Input: part model. Units: mm. Frame: model coordinates. A direction names the side the tool comes from. Coordinates: 2 decimals unless noted, no trailing zeros. Order: outer loops, then holes, each group sorted by start corner. A loop starts at its lowest first (then second) coordinate and runs counter-clockwise, first axis right, second up. Notation, with made-up numbers: M 38.5,74 L 96.5,74 A16 ccw 96.5,78 Z; hole C 17,2.5 d8. An arc over 180 degrees is marked long. One line per item, written item: value.
```python
from build123d import *

# Parameters (mm, degrees)
BOSS_EXTRUDE2_DEPTH   = 2.5
BOSS_EXTRUDE2_2_DEPTH = 2.5
BOSS_EXTRUDE2_3_DEPTH = 2.5
BOSS_EXTRUDE2_4_DEPTH = 2.5
BOSS_EXTRUDE3_DEPTH   = 1.5
SKETCH1_W             = 10
SKETCH1_H             = 10
BOSS_EXTRUDE4_DEPTH   = 2.8
CUT_EXTRUDE11_DEPTH   = 1
CUT_EXTRUDE14_DEPTH   = 1


with BuildPart() as part:
    # Sketch2 → Boss-Extrude2 (new body)
    with BuildSketch(Plane(origin=(0, 0, 0), x_dir=(1, 0, 0), z_dir=(0, 1, 0))):
        Polygon((-2, 6), (-6, 6), (-6, 2), (-5, 2), (-5, 5), (-2, 5), align=None)
    extrude(amount=BOSS_EXTRUDE2_DEPTH)



with BuildPart() as body_2:
    # Sketch2 → Boss-Extrude2 2 (new body)
    with BuildSketch(Plane(origin=(0, 0, 0), x_dir=(1, 0, 0), z_dir=(0, 1, 0))):
        Polygon((2, 6), (2, 5), (5, 5), (5, 2), (6, 2), (6, 6), align=None)
    extrude(amount=BOSS_EXTRUDE2_2_DEPTH)


with BuildPart() as body_3:
    # Sketch2 → Boss-Extrude2 3 (new body)
    with BuildSketch(Plane(origin=(0, 0, 0), x_dir=(1, 0, 0), z_dir=(0, 1, 0))):
        Polygon((5, -2), (5, -5), (2, -5), (2, -6), (6, -6), (6, -2), align=None)
    extrude(amount=BOSS_EXTRUDE2_3_DEPTH)


with BuildPart() as body_4:
    # Sketch2 → Boss-Extrude2 4 (new body)
    with BuildSketch(Plane(origin=(0, 0, 0), x_dir=(1, 0, 0), z_dir=(0, 1, 0))):
        Polygon((-6, -2), (-5, -2), (-5, -5), (-2, -5), (-2, -6), (-6, -6), align=None)
    extrude(amount=BOSS_EXTRUDE2_4_DEPTH)

    # Sketch2<4> → Boss-Extrude3 (add)
    with BuildSketch(Plane(origin=(0, 0, 0), x_dir=(1, 0, 0), z_dir=(0, 1, 0))):
        Polygon((-2, 6), (-6, 6), (-6, 2), (-5, 2), (-5, 5), (-2, 5), align=None)
        Polygon((2, 6), (2, 5), (5, 5), (5, 2), (6, 2), (6, 6), align=None)
        Polygon((5, -2), (5, -5), (2, -5), (2, -6), (6, -6), (6, -2), align=None)
        Polygon((-6, -2), (-5, -2), (-5, -5), (-2, -5), (-2, -6), (-6, -6), align=None)
    extrude(amount=-BOSS_EXTRUDE3_DEPTH)


with BuildPart() as boss_extrude3_piece_1:
    # of the separate pieces the step leaves, piece 1, a body of its own (boss_extrude3_pieces)
    add(body_4.part.solids().sort_by_distance((-6, 2.5, 2))[0])


with BuildPart() as boss_extrude3_piece_2:
    # of the separate pieces the step leaves, piece 2, a body of its own (boss_extrude3_pieces)
    add(body_4.part.solids().sort_by_distance((-2, 0, -6))[0])


with BuildPart() as boss_extrude3_piece_3:
    # of the separate pieces the step leaves, piece 3, a body of its own (boss_extrude3_pieces)
    add(body_4.part.solids().sort_by_distance((2, 0, -6))[0])


with BuildPart() as boss_extrude3_piece_4:
    # of the separate pieces the step leaves, piece 4, a body of its own (boss_extrude3_pieces)
    add(body_4.part.solids().sort_by_distance((5, 0, 2))[0])


with BuildPart() as part_1:
    add(part.part)

    add(body_2.part)  # Boss-Extrude4 merges body 2

    add(body_3.part)  # Boss-Extrude4 merges body 3

    add(boss_extrude3_piece_1.part)  # Boss-Extrude4 merges Boss-Extrude3 piece 1

    add(boss_extrude3_piece_2.part)  # Boss-Extrude4 merges Boss-Extrude3 piece 2

    add(boss_extrude3_piece_3.part)  # Boss-Extrude4 merges Boss-Extrude3 piece 3

    add(boss_extrude3_piece_4.part)  # Boss-Extrude4 merges Boss-Extrude3 piece 4
    # Sketch1 → Boss-Extrude4 (add)
    with BuildSketch(Plane(origin=(0, 0, 0), x_dir=(1, 0, 0), z_dir=(0, 1, 0))):
        Rectangle(SKETCH1_W, SKETCH1_H)
        with BuildLine():
            ThreePointArc((1.617598637, -1.615265837), (3.065, 0), (1.617598637, 1.615265837))
            ThreePointArc((1.617598637, 1.615265837), (1.474163525, 1.620673027), (1.331431871, 1.605489361))
            Line((1.331431871, 1.605489361), (-1.677221968, 1.064808042))
            ThreePointArc((-1.677221968, 1.064808042), (-1.895132853, 0.999347796), (-2.092605578, 0.886322491))
            ThreePointArc((-2.092605578, 0.886322491), (-2.54112078, 0), (-2.092605578, -0.886322491))
            ThreePointArc((-2.092605578, -0.886322491), (-1.895132853, -0.999347796), (-1.677221968, -1.064808042))
            Line((-1.677221968, -1.064808042), (1.331431871, -1.605489361))
            ThreePointArc((1.331431871, -1.605489361), (1.474163525, -1.620673027), (1.617598637, -1.615265837))
        make_face(mode=Mode.SUBTRACT)
    extrude(amount=BOSS_EXTRUDE4_DEPTH)

    # 3DSketch1 → Cut-Extrude11 (cut, along a direction that is not the sketch's normal)
    with BuildSketch(Plane(origin=(5, 2.8, 5), x_dir=(-0.693702510890827, -0.1937876486453734, -0.6937025108908424), z_dir=(0.7071067811865555, 0, -0.7071067811865397))):
        Polygon((0, 0), (-0.732362778, 3.707562105), (7.206933902, 0), align=None)
    extrude(amount=-CUT_EXTRUDE11_DEPTH, dir=(1, 0, 0), mode=Mode.SUBTRACT)

    # 3DSketch1<9> → Cut-Extrude14 (cut, along a direction that is not the sketch's normal)
    with BuildSketch(Plane(origin=(5, 2.8, 5), x_dir=(-0.693702510890827, -0.1937876486453734, -0.6937025108908424), z_dir=(0.7071067811865555, 0, -0.7071067811865397))):
        Polygon((0, 0), (-0.732362778, 3.707562105), (7.206933902, 0), align=None)
    extrude(amount=CUT_EXTRUDE14_DEPTH, dir=(0, 0, -1), mode=Mode.SUBTRACT)


solid = part_1.part
```
(1) Cut plane A-A on y = 0.5. Output: boundary loops of the cut face in (x, z) (3 decimals).
Data:
outline: M -6,-6 L -2,-6 L -2,-5 L 2,-5 L 2,-6 L 6,-6 L 6,-2 L 5,-2 L 5,2 L 6,2 L 6,6 L 2,6 L 2,5 L -2,5 L -2,6 L -6,6 L -6,2 L -5,2 L -5,-2 L -6,-2 Z; hole M -2.093,-0.886 A1 ccw -1.677,-1.065 L 1.331,-1.605 A1 ccw 1.618,-1.615 A1.625 ccw 1.618,1.615 A1 ccw 1.331,1.605 L -1.677,1.065 A1 ccw -2.093,0.886 A1.1 ccw Z
(2) First-contact query: pin 1 (5 mm diameter, centred on x = 2, z = -0.5, fed in from -Y). Flat tip, straight axial feed; report the tip coordinate or a pass-through.
Data:
pin 1: stops at y = 0
(3) Cut plane C-C on y = -0.45. Output: boundary loops of the cut face in (x, z), plus the area to 3 significant figures.
Data:
outline: M -6,-6 L -2,-6 L -2,-5 L -5,-5 L -5,-2 L -6,-2 Z; M -6,2 L -5,2 L -5,5 L -2,5 L -2,6 L -6,6 Z; M 2,-6 L 6,-6 L 6,-2 L 5,-2 L 5,-5 L 2,-5 Z; M 2,5 L 5,5 L 5,2 L 6,2 L 6,6 L 2,6 Z
area: 28.0 mm2
(4) Draft query along Z for faces 1 (the flat face through (4, 1, -6)), 2 (the flat face through (2.699, 2.295, 3.192)), 3 (the flat face through (-4.9, -1.5, 5.3)), 4 (the flat face through (3.3, 2.6, 2.3)). Return one class per face: released by +Z, released by -Z, zero draft, split by the parting line, or undercut.
Data:
face 1: released by -Z
face 2: undercut
face 3: zero draft
face 4: undercut
(5) Ray query, line 1 (X direction, y = -0.55, z = -4); line 2 (Z direction, x = 5.25, y = 0.05). Return the intervals inside material, ascending. Write a range as from..to.
Data:
line 1: x = -6..-5, 5..6
line 2: z = -6..-2, 2..6
(6) Access query for faces 5 (the flat face through (2, 0.5, -5.5)), 6 (the flat face through (-0.194, 1.38, 1.331)), 7 (the flat face through (5.5, 0.5, -2)), 8 (the flat face through (3, -1, -5)), 9 (the flat face through (-5.5, 0.5, 2)). Directions: +Z, -Z, +X, -X, +Y, -Y. A direction counts if a zero-diameter tool reaches every point of the face in a straight line with its end or side. Return the directions, or none.
Data:
face 5: -Z, +Y, -Y
face 6: +Y, -Y
face 7: +X, +Y, -Y
face 8: -Y
face 9: -X, +Y, -Y
(7) Cut plane D-D on x = -4.5. Output: boundary loops of the cut face in (y, z).
Data:
outline: M -1.5,-6 L 2.5,-6 L 2.5,-5 L 2.8,-5 L 2.8,5 L 2.5,5 L 2.5,6 L -1.5,6 L -1.5,5 L 0,5 L 0,-5 L -1.5,-5 Z
(8) Cut plane B-B on x = 0. Output: boundary loops of the cut face in (y, z), plus the area to 3 significant figures.
Data:
outline: M 0,-5 L 2.8,-5 L 2.8,-1.37 L 0,-1.37 Z; M 0,1.37 L 2.8,1.37 L 2.8,5 L 0,5 Z
area: 20.3 mm2
